The figure shows three views and two pictorial views of one solid part (mm, origin at its lowest corner). Answer the questions. A direction names the side the tool comes from. Coordinates: 2 decimals unless noted, no trailing zeros. Loops run counter-clockwise (first coordinate to the right, second up) from the corner with the lowest first, then second, coordinate; pieces in that order, holes last. Notation, with made-up numbers: (66, 27) - (99, 27) arc R30 ccw to (99, 53) - close; hole circle Ø2 at (-24.5, 62.5). An arc over 180 degrees is marked (long way). Write each question's results on one line, items separated by ' | '. Start each with the question number.
Item 1: Section D-D, the plane x = 17 is taken. Write down the section's boundary in (y, z).
Item 2: Consider probe 1 along Y at (x, z) = (28, 57); probe 2 along X at (y, z) = (33.5, 56); probe 3 along Z at (x, y) = (43.5, 47.5). Determine where each line is inside the solid, lowest interval first. Write a range as [from, to].
Item 3: Section B-B, the plane y = 39 is taken. Write down the section's boundary in (x, z).
Item 4: Section A-A, the plane x = 31.5 is taken. Write down the section's boundary in (y, z).
Item 5: A tool of negligible diameter and unlimited length cuts with its end or side. For the marked faces 5, 6 and 7, from which of +Z, -Z, +X, -X, +Y, -Y can it reach the whole face along a straight path? Write none if from no direction.
Item 6: Each of these flat-tipped pins is pushed along its axis until it touches: pin 1 Ø7.5 at (y, z) = (24.5, 57) entering from -X; pin 2 Ø7.5 at (y, z) = (28.5, 57) entering from +X; pin 3 Ø16.5 at (x, z) = (33, 58.5) entering from -Y. Where does it stop, or does it pass through?
Item 7: For a pull along X with two mould halves and no side action, classify the marked faces 1, 2, 3 and 4 as +X half, -X half, draft (parallel to the pull), parting line (faces both ways), or undercut.
Item 8: Section C-C, the plane z = 53.5 is taken. Write down the section's boundary in (x, y), plus the area to 3 significant figures.
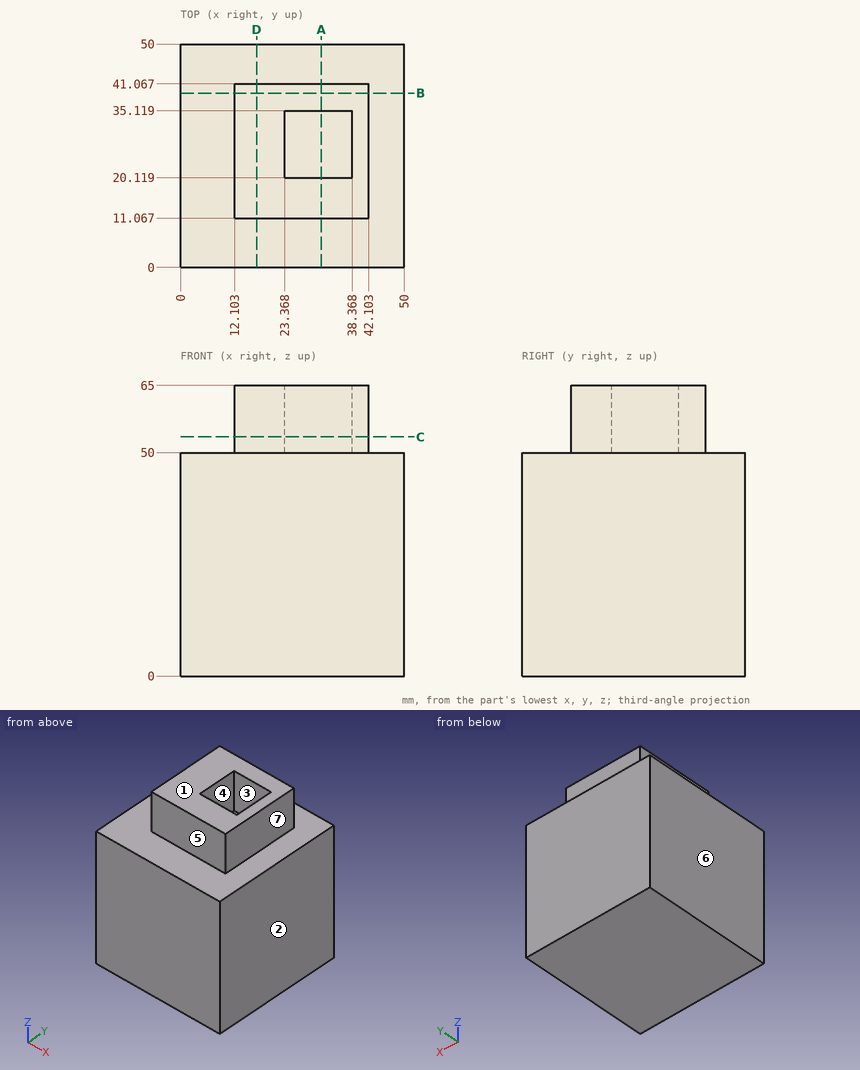
Answer key:
1) outline: (0, 0) - (50, 0) - (50, 50) - (41.07, 50) - (41.07, 65) - (11.07, 65) - (11.07, 50) - (0, 50) - close
2) probe 1: y = [11.07, 20.12], [35.12, 41.07] | probe 2: x = [12.1, 23.37], [38.37, 42.1] | probe 3: z = [0, 50]
3) outline: (0, 0) - (50, 0) - (50, 50) - (42.1, 50) - (42.1, 65) - (12.1, 65) - (12.1, 50) - (0, 50) - close
4) outline: (0, 0) - (50, 0) - (50, 50) - (41.07, 50) - (41.07, 65) - (35.12, 65) - (35.12, 50) - (20.12, 50) - (20.12, 65) - (11.07, 65) - (11.07, 50) - (0, 50) - close
5) face 5: +Z, +X, -X, -Y | face 6: +Z, -Z, -X, +Y, -Y | face 7: +Z, +X, +Y, -Y
6) pin 1: stops at x = 12.1 | pin 2: stops at x = 42.1 | pin 3: stops at y = 11.07
7) face 1: draft | face 2: +X half | face 3: undercut | face 4: undercut
8) outline: (12.1, 11.07) - (42.1, 11.07) - (42.1, 41.07) - (12.1, 41.07) - close; hole (23.37, 20.12) - (38.37, 20.12) - (38.37, 35.12) - (23.37, 35.12) - close | area: 675 mm^2
